Study the drawing (mm; zero at the part's minimum x, y, z) and answer. A direction names the side the tool comes from. Round coordinates to 2 decimals unless told otherwise and drop trailing zeros. Write each loop counter-clockwise with the first axis right and the second up, starting at its lowest first coordinate (ties: lowest second). Pieces come first, ordered by that corner, then holes.
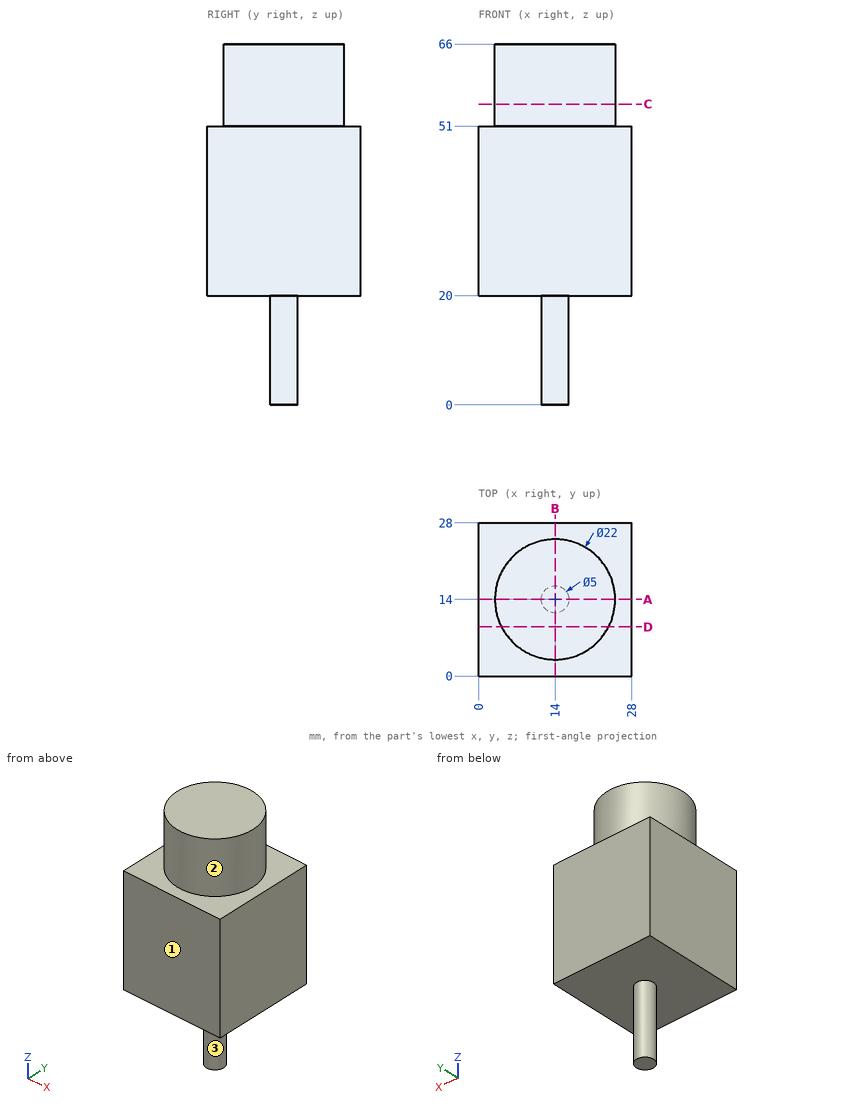
1. Section A-A on y = 14 is taken. Determine the outline of the cut face in (x, z), plus the area to 3 significant figures.
Geometry says:
outline: (0, 20) - (11.5, 20) - (11.5, 0) - (16.5, 0) - (16.5, 20) - (28, 20) - (28, 51) - (25, 51) - (25, 66) - (3, 66) - (3, 51) - (0, 51) - close
area: 1,300 mm2
2. Given pin 1 (1.5 mm diameter, centred on x = 6.5, z = 53, fed in from +Y), flat-ended and moving along its own axis, determine where the tip first touches the part or whether it passes through.
Geometry says:
pin 1: stops at y = 22.69
3. Straight lines are drawn through the part: line 1 along Z through (x, y) = (25.5, 2.5); line 2 along Z through (x, y) = (12.5, 4.25); line 3 along Y through (x, z) = (23.75, 63). For each, find the intervals that lie inside material, in ascending order.
Geometry says:
line 1: z = 20 to 51
line 2: z = 20 to 66
line 3: y = 8.91 to 19.09
4. Section C-C on z = 55 is taken. Determine the outline of the cut face in (x, y).
Geometry says:
outline: circle Ø22 at (14, 14)
5. A tool of negligible diameter and unlimited length cuts with its end or side. For the marked faces 1, 2 and 3, from which of +Z, -Z, +X, -X, +Y, -Y can it reach the whole face along a straight path? Write none if from no direction.
Geometry says:
face 1: +Z, -Z, +X, -X, -Y
face 2: +Z
face 3: -Z
6. Section D-D on y = 9 is taken. Determine the outline of the cut face in (x, z), plus the area to 3 significant figures.
Geometry says:
outline: (0, 20) - (28, 20) - (28, 51) - (23.8, 51) - (23.8, 66) - (4.2, 66) - (4.2, 51) - (0, 51) - close
area: 1,160 mm2
